The figure shows three views and two pictorial views of one solid part (mm, origin at its lowest corner). Answer the questions. A direction names the side the tool comes from. Round coordinates to 2 decimals unless told otherwise and drop trailing zeros. Loops run counter-clockwise (first coordinate to the right, second up) from the corner with the lowest first, then second, coordinate; pieces in that order, holes last. Notation, with made-up numbers: (32, 54) - (88, 54) arc R32 cw to (88, 93) - close; hole circle Ø5 at (41, 89.25). An arc over 180 degrees is marked (long way). Use one line per item in the form item = value. Start each with the question number.
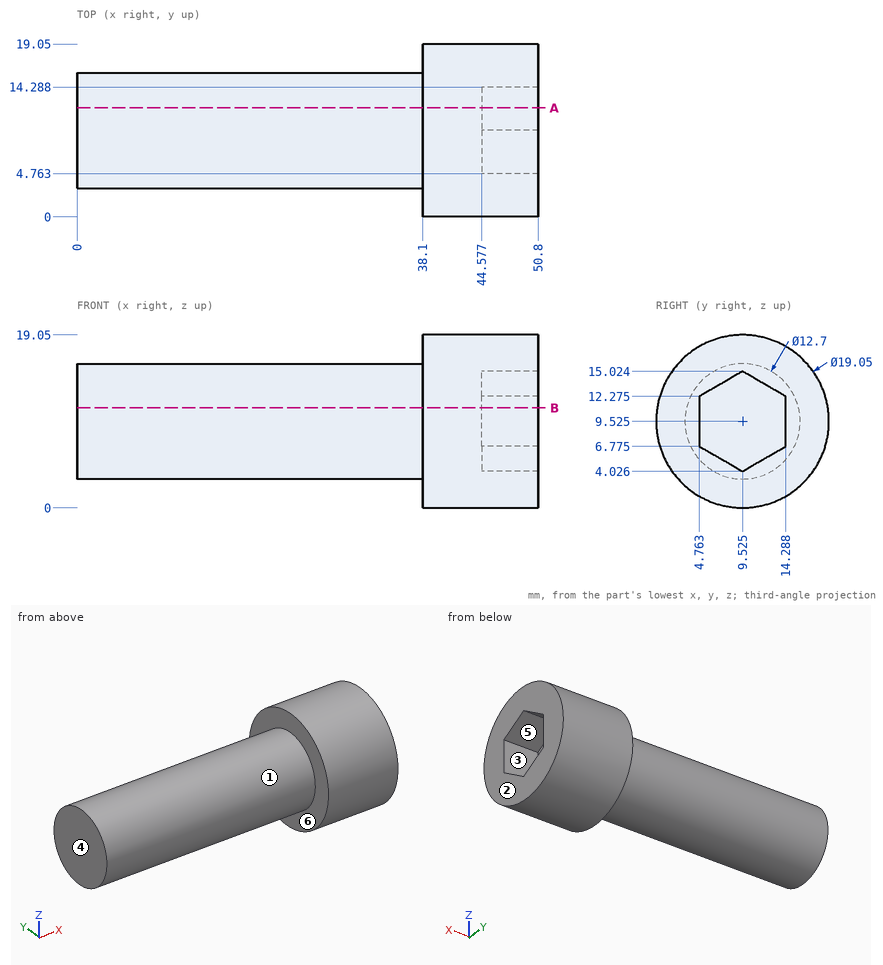
1) For the marked faces 4, 5 and 6, determine the directions among +Z, -Z, +X, -X, +Y, -Y from which every point of the face is accessible in a straight line to the end or side of a thin tool.
2) Determine the mould class of the marked faces 1, 2 and 3 for opening direction Z: +Z half, -Z half, draft (parallel to the pull), parting line (faces both ways), or undercut.
3) A cutting plane is placed at A-A on y = 12. Write down the section's boundary in (x, z) (1 decimal).
4) Straight lines are drawn through the part: line 1 (Y direction, x = 46, z = 8.75); line 2 (Y direction, x = 17, z = 9.5) (1 decimal); line 3 (X direction, y = 3.5, z = 6.75). For each, find the intervals that lie inside material, in ascending order. Write a range as from..to.
5) Flat-ended cylindrical pins translate along their axes: pin 1 (6 mm diameter, centred on x = 28, y = 9.5, fed in from +Z) (1 decimal); pin 2 (10 mm diameter, centred on x = 13, z = 8.5, fed in from +Y) (1 decimal); pin 3 (1 mm diameter, centred on y = 2, z = 11.5, fed in from -X). Find the tip coordinate at first contact, or state that the pin passes through.
6) A cutting plane is placed at B-B on z = 11. Write down the section's boundary in (x, y) (1 decimal).
Checks:
q1.face_4 = +Z, -Z, -X, +Y, -Y
q1.face_5 = +X
q1.face_6 = -X
q2.face_1 = parting line
q2.face_2 = draft
q2.face_3 = undercut
q3.outline = (0, 3.7) - (38.1, 3.7) - (38.1, 0.3) - (50.8, 0.3) - (50.8, 5.5) - (44.6, 5.5) - (44.6, 13.6) - (50.8, 13.6) - (50.8, 18.7) - (38.1, 18.7) - (38.1, 15.4) - (0, 15.4) - close
q4.line_1 = 0.03..4.76, 14.29..19.02
q4.line_2 = 3.2..15.9
q4.line_3 = 38.1..50.8
q5.pin_1 = 15.9
q5.pin_2 = 15.9
q5.pin_3 = 38.1
q6.outline = (0, 3.3) - (38.1, 3.3) - (38.1, 0.1) - (50.8, 0.1) - (50.8, 4.8) - (44.6, 4.8) - (44.6, 14.3) - (50.8, 14.3) - (50.8, 18.9) - (38.1, 18.9) - (38.1, 15.7) - (0, 15.7) - close
